Autodesk Inventor part; units mm, degrees
ref_plane "YZ Plane" through (0, 0, 0) normal (1, 0, 0) x (0, 1, 0)
ref_plane "XZ Plane" through (0, 0, 0) normal (0, 1, 0) x (-1, 0, 0)
ref_plane "XY Plane" through (0, 0, 0) normal (0, 0, 1) x (1, 0, 0)
sketch "Sketch1" plane through (0, 0, 0) normal (0, 0, 1) x (1, 0, 0)
  circle A0 centre (0, 0) radius 54.5
  line L0 (-100, 100) -> (100, 100)
  line L1 (100, 100) -> (100, -100)
  line L2 (100, -100) -> (-100, -100)
  line L3 (-100, -100) -> (-100, 100)
  dimension "d0" = 109
  dimension "d3" = 200
  dimension "d4" = 200
extrude "Extrusion1" add sketch "Sketch1" along normal blind 2
sketch "Sketch2" plane through (0, 0, 2) normal (0, 0, 1) x (1, 0, 0)
  circle A0 centre (0, 65) radius 3
  circle A1 centre (-56.2917, 32.5) radius 3
  circle A2 centre (-56.2917, -32.5) radius 3
  circle A3 centre (0, -65) radius 3
  circle A4 centre (56.2917, -32.5) radius 3
  circle A5 centre (56.2917, 32.5) radius 3
  circle A6 centre (0, 0) radius 65
  dimension "d8" = 6
  dimension "d11" = 360
extrude "Extrusion2" cut sketch "Sketch2" against normal blind 2 contours A0 A6 | A6 A0 | A6 A1 | A1 A6 | A6 A5 | A5 A6 | A6 A2 | A2 A6 | A6 A4 | A4 A6 | A6 A3 | A3 A6
properties part number "uppe sheet"
Design review of the part built by this model. Coordinates are the model's own, in mm. Coordinates: 2 decimals unless noted, no trailing zeros. Order: outer loops, then holes, each group sorted by start corner. A loop starts at its lowest first (then second) coordinate and runs counter-clockwise, first axis right, second up.
1) Take a section at D-D, the plane y = 32.5. Give the boundary of the cut face in (x, z).
2) Wall thickness on line 1 along Y through (x, z) = (0, 1.55); line 2 along X through (y, z) = (65, 0.5); line 3 along X through (y, z) = (-32.5, 1.2): over which ranges is each line inside the solid? List them lowest first.
3) Take a section at C-C, the plane x = 0. Give the boundary of the cut face in (y, z).
4) Take a section at A-A, the plane y = 0. Give the boundary of the cut face in (x, z).
5) Take a section at B-B, the plane z = 0.85. Give the boundary of the cut face in (x, y).
6) Mouldability with a two-part tool opening along Y and no side actions: class faces 1 (the flat face through (-46, 46, 0)), 2 (the cylindrical face through (-53.43, 33.4, 1.01)) as +Y half, -Y half, draft (parallel to the pull), parting line (faces both ways), or undercut.
Returned:
1. outline: (-100, 0) - (-59.29, 0) - (-59.29, 2) - (-100, 2) - close; (-53.29, 0) - (-43.75, 0) - (-43.75, 2) - (-53.29, 2) - close; (43.75, 0) - (53.29, 0) - (53.29, 2) - (43.75, 2) - close; (59.29, 0) - (100, 0) - (100, 2) - (59.29, 2) - close
2. line 1: y = -100 to -68, -62 to -54.5, 54.5 to 62, 68 to 100
2. line 2: x = -100 to -3, 3 to 100
2. line 3: x = -100 to -59.29, -53.29 to -43.75, 43.75 to 53.29, 59.29 to 100
3. outline: (-100, 0) - (-68, 0) - (-68, 2) - (-100, 2) - close; (-62, 0) - (-54.5, 0) - (-54.5, 2) - (-62, 2) - close; (54.5, 0) - (62, 0) - (62, 2) - (54.5, 2) - close; (68, 0) - (100, 0) - (100, 2) - (68, 2) - close
4. outline: (-100, 0) - (-54.5, 0) - (-54.5, 2) - (-100, 2) - close; (54.5, 0) - (100, 0) - (100, 2) - (54.5, 2) - close
5. outline: (-100, -100) - (100, -100) - (100, 100) - (-100, 100) - close; hole circle Ø6 at (-56.29, -32.5); hole circle Ø6 at (-56.29, 32.5); hole circle Ø109 at (0, 0); hole circle Ø6 at (0, -65); hole circle Ø6 at (0, 65); hole circle Ø6 at (56.29, -32.5); hole circle Ø6 at (56.29, 32.5)
6. face 1: draft
6. face 2: undercut
